Can you work these out from the model? Positions are in its coordinate system, mm. A direction names the side the tool comes from. Round coordinates to 2 decimals unless told otherwise and drop trailing zeros. Write each loop counter-clockwise with the first axis right and the second up, starting at its lowest first coordinate (ties: lowest second). Pieces come first, ordered by that corner, then holes. Notation, with made-up numbers: (70.5, 15.25) -> (86.5, 15.25) arc R26 cw to (86.5, 52.25) -> close; hole circle Ø4 at (42, -5). An arc over 180 degrees is marked (long way). Write item = value, one per line. Start each with the question number.
1) If I drill on line 1 (Y direction, x = -2, z = -2.5); line 2 (Y direction, x = -1, z = -2) (3 decimals); line 3 (Z direction, x = 1.25, y = 4.5), over which ranges is the centre line in solid material (lowest first)?
2) Imagine slicing it at C-C, the plane y = -6. Please give me the cut outline in (x, z).
3) Thinking about a two-plate mould opening in Z: for faces 4 (the face through (-2, 6.35, -2)), 5 (the face through (2.604, -13.086, -0.82)), 6 (the face through (0, 3.175, 0)), 7 (the face through (-2.25, 4.78, 0.78)), which applies, +Z half, -Z half, draft (parallel to the pull), parting line (faces both ways), or undercut?
4) Imagine slicing it at D-D, the plane z = -4. Please give me the cut outline in (x, y), then the cut area to 3 significant figures.
5) For faces 1 (the face through (-4.153, 3.131, 1.722)), 2 (the face through (0, 0, -3)), 3 (the face through (-0.45, 4.78, 2.34)), which set-ups out of +Z, -Z, +X, -X, +Y, -Y let a thin tool reach every point of the face, with its end or its side?
6) Imagine slicing it at A-A, the plane z = 1.5. Please give me the cut outline in (x, y) (3 decimals).
7) Imagine slicing it at B-B, the plane x = -0.25. Please give me the cut outline in (y, z) (3 decimals), then the cut area to 3 significant figures.
8) I'm going to push flat-ended pins straight in: pin 1 (5 mm diameter, centred on x = 3, z = -1.5, fed in from -Y); pin 2 (1 mm diameter, centred on x = 1, y = -11, fed in from -Z); pin 3 (5 mm diameter, centred on x = 1.5, y = -16, fed in from +Z). Where does each tip first touch, or does it pass through?
Autodesk Inventor part; units mm, degrees
ref_plane "YZ Plane" through (0, 0, 0) normal (1, 0, 0) x (0, 1, 0)
ref_plane "XZ Plane" through (0, 0, 0) normal (0, 1, 0) x (-1, 0, 0)
ref_plane "XY Plane" through (0, 0, 0) normal (0, 0, 1) x (1, 0, 0)
sketch "Sketch1" plane through (0, 0, 0) normal (0, 1, 0) x (-1, 0, 0)
  circle A0 centre (0, 0) radius 4.4958
  dimension "d0" = 8.9916
extrude "Extrusion1" add sketch "Sketch1" along normal blind 6.35
sketch "Sketch2" plane through (0, 0, 0) normal (0, -1, 0) x (1, 0, 0)
  point P0 (0, 0)
sketch "Sketch4" plane through (0, 6.35, 0) normal (0, 1, 0) x (1, 0, 0)
  circle A0 centre (0, 0) radius 4.4958
  line L0 (-0.8834, 2.6038) -> (1.8133, 2.067)
  line L1 (1.8133, 2.067) -> (2.6967, -0.5368)
  line L2 (2.6967, -0.5368) -> (0.8834, -2.6038)
  line L3 (0.8834, -2.6038) -> (-1.8133, -2.067)
  line L4 (-1.8133, -2.067) -> (-2.6967, 0.5368)
  line L5 (-2.6967, 0.5368) -> (-0.8834, 2.6038)
  dimension "d4" = 4.7625
extrude "Extrusion2" cut sketch "Sketch4" against normal blind 3.175 contours L0 L1 L2 L3 L4 L5
sketch "Sketch5" plane through (0, 0, 0) normal (0, -1, 0) x (1, 0, 0)
  circle A0 centre (0, 0) radius 4.4958
  circle A1 centre (0, 0) radius 2.7305
  dimension "d7" = 5.461
extrude "Extrusion3" add sketch "Sketch5" along normal blind 26.543 contours A1
thread "Thread1"
properties part number "WheelBracketScrew"
Reported:
q1.line_1 = 0 to 6.35
q1.line_2 = -26.543 to 3.175
q1.line_3 = -4.32 to -2.18, 2.19 to 4.32
q2.outline = circle Ø5.46 at (0, 0)
q3.face_4 = draft
q3.face_5 = parting line
q3.face_6 = undercut
q3.face_7 = undercut
q4.outline = (-2.05, 0) -> (2.05, 0) -> (2.05, 6.35) -> (-2.05, 6.35) -> close
q4.area = 26.1 mm²
q5.face_1 = +Y, -Y
q5.face_2 = -Y
q5.face_3 = +Y
q6.outline = (-4.238, 0) -> (-2.282, 0) -> (-2.282, -26.543) -> (2.282, -26.543) -> (2.282, 0) -> (4.238, 0) -> (4.238, 6.35) -> (1.852, 6.35) -> (1.852, 3.175) -> (-2.006, 3.175) -> (-2.006, 6.35) -> (-4.238, 6.35) -> close
q7.outline = (-26.543, -2.719) -> (0, -2.719) -> (0, -4.489) -> (6.35, -4.489) -> (6.35, -2.478) -> (3.175, -2.478) -> (3.175, 2.378) -> (6.35, 2.378) -> (6.35, 4.489) -> (0, 4.489) -> (0, 2.719) -> (-26.543, 2.719) -> close
q7.area = 186 mm²
q8.pin_1 = -26.54
q8.pin_2 = -2.68
q8.pin_3 = 2.73
